Geometry check sheet. Reference: the model listing, model coordinates, mm. Face numbers are marked on the shaded views. Coordinates: 2 decimals unless noted, no trailing zeros. Order: outer loops, then holes, each group sorted by start corner. A loop starts at its lowest first (then second) coordinate and runs counter-clockwise, first axis right, second up. Notation, with made-up numbers: M -31,16.5 L -7,16.5 A27 cw -7,47.5 Z; hole C -9,-20 d5. An arc over 180 degrees is marked long. One line per item, written item: value. Start each with the question number.
1) Draft check along Y on the marked faces 1 and 2. Enter one of: pulls with the +Y half, pulls with the -Y half, needs draft (parallel to the pull), parting line crosses it, or undercut.
2) Sectioned sample at B-B, the plane x = 4. Enter the section's corners in (y, z) (3 decimals), then the cut area to 3 significant figures.
3) Sectioned sample at A-A, the plane y = 1.9. Enter the section's corners in (x, z) (3 decimals).
4) Go/stop test with flat-tipped pins: P1, Ø1.6, axis at y = 1, z = -73.5, coming from the -X side (3 decimals); P2, Ø1.6, axis at y = 1.5, z = 72.5, coming from the +X side (3 decimals). Record where each tip stops, or that it passes through.
5) Thickness scan on L1, parallel to Z at x = 36.5, y = 1.55. Record the ranges inside material, lowest first. Write a range as from..to.
```python
from build123d import *

# Parameters (mm, degrees)
SKETCH1_W           = 82.55
SKETCH1_H           = 152.4
BOSS_EXTRUDE1_DEPTH = 3.175
SKETCH2_W           = 6.35
SKETCH2_H           = 6.35
SKETCH2_W_2         = 9.525
CUT_EXTRUDE1_DEPTH  = 4.175


with BuildPart() as part:
    # Sketch1 → Boss-Extrude1 (new body)
    with BuildSketch(Plane(origin=(0, 0, 0), x_dir=(1, 0, 0), z_dir=(0, 1, 0))):
        Rectangle(SKETCH1_W, SKETCH1_H)
    extrude(amount=BOSS_EXTRUDE1_DEPTH)

    # Sketch2 → Cut-Extrude1 (cut, through all)
    with BuildSketch(Plane(origin=(0, 3.175, 0), x_dir=(1, 0, 0), z_dir=(0, 1, 0))):
        with Locations((-38.1, -73.025)):
            Rectangle(SKETCH2_W, SKETCH2_H)
        with Locations((-4.7625, -73.025)):
            Rectangle(SKETCH2_W_2, SKETCH2_H)
        with Locations((4.7625, -73.025)):
            Rectangle(SKETCH2_W_2, SKETCH2_H)
        with Locations((38.1, -73.025)):
            Rectangle(SKETCH2_W, SKETCH2_H)
    cut_extrude1 = extrude(amount=-CUT_EXTRUDE1_DEPTH, mode=Mode.SUBTRACT)

    # Mirror1: Cut-Extrude1 across plane
    add(cut_extrude1.mirror(Plane.XY), mode=Mode.SUBTRACT)


solid = part.part
```
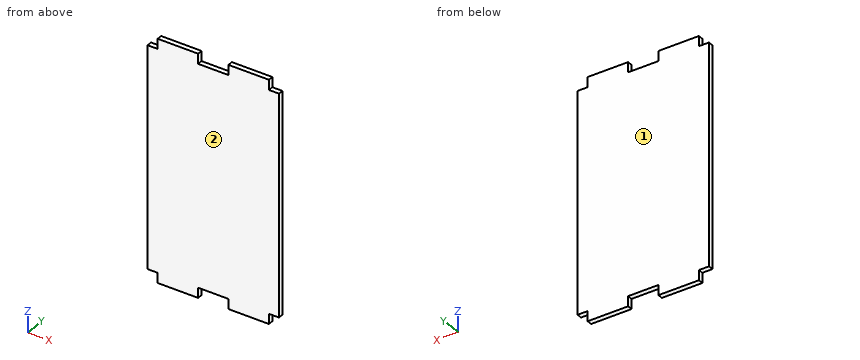
Final values:
1. face 1: pulls with the +Y half
1. face 2: pulls with the -Y half
2. outline: M 0,-69.85 L 3.175,-69.85 L 3.175,69.85 L 0,69.85 Z
2. area: 444 mm^2
3. outline: M -41.275,-69.85 L -34.925,-69.85 L -34.925,-76.2 L -9.525,-76.2 L -9.525,-69.85 L 9.525,-69.85 L 9.525,-76.2 L 34.925,-76.2 L 34.925,-69.85 L 41.275,-69.85 L 41.275,69.85 L 34.925,69.85 L 34.925,76.2 L 9.525,76.2 L 9.525,69.85 L -9.525,69.85 L -9.525,76.2 L -34.925,76.2 L -34.925,69.85 L -41.275,69.85 Z
4. P1: stops at x = -34.925
4. P2: stops at x = 34.925
5. L1: z = -69.85..69.85
